```python
from build123d import *

# Parameters (mm, degrees)
SKETCH1_W           = 40
SKETCH1_H           = 40
BOSS_EXTRUDE1_DEPTH = 5
FILLET1_R           = 5
SKETCH2_R           = 15
BOSS_EXTRUDE2_DEPTH = 2.5
SKETCH3_R           = 3
BOSS_EXTRUDE3_DEPTH = 22.5
BOSS_EXTRUDE5_DEPTH = 82
CHAMFER1_SIZE       = 0.5
SKETCH5_R           = 2.15
CUT_EXTRUDE1_DEPTH  = 10
SKETCH6_W           = 8.611155486
SKETCH6_H           = 40
BOSS_EXTRUDE6_DEPTH = 12
CHAMFER2_SIZE       = 5


with BuildPart() as part:
    # Sketch1 → Boss-Extrude1 (new body)
    with BuildSketch(Plane.XY):
        Rectangle(SKETCH1_W, SKETCH1_H)
    extrude(amount=BOSS_EXTRUDE1_DEPTH)

    # Fillet1
    fillet1_edges = [part.edges().sort_by_distance(p)[0] for p in [
        (20, -20, 2.5),
        (-20, -20, 2.5),
        (-20, 20, 2.5),
        (20, 20, 2.5),
    ]]
    fillet(fillet1_edges, radius=FILLET1_R)

    # Sketch2 → Boss-Extrude2 (add)
    with BuildSketch(Plane.XY.offset(5)):
        Circle(SKETCH2_R)
    extrude(amount=BOSS_EXTRUDE2_DEPTH)

    # Sketch3 → Boss-Extrude3 (add)
    with BuildSketch(Plane.XY.offset(7.5)):
        with Locations(Location((0, 0, 0), (0, 0, 180))):
            Circle(SKETCH3_R)
    extrude(amount=BOSS_EXTRUDE3_DEPTH)

    # Sketch4 → Boss-Extrude5 (add)
    with BuildSketch(Plane(origin=(0, 0, 0), x_dir=(-1, 0, 0), z_dir=(0, 0, -1))):
        with BuildLine():
            Line((-20, -15), (-20, 15))
            ThreePointArc((-20, 15), (-18.535533906, 18.535533906), (-15, 20))
            Line((-15, 20), (15, 20))
            ThreePointArc((15, 20), (18.535533906, 18.535533906), (20, 15))
            Line((20, 15), (20, -15))
            ThreePointArc((20, -15), (18.535533906, -18.535533906), (15, -20))
            Line((15, -20), (-15, -20))
            ThreePointArc((-15, -20), (-18.535533906, -18.535533906), (-20, -15))
        make_face()
    extrude(amount=BOSS_EXTRUDE5_DEPTH)

    # Chamfer1
    chamfer1_edges = [part.edges().sort_by_distance(p)[0] for p in [
        (3, 0, 30),
    ]]
    chamfer(chamfer1_edges, length=CHAMFER1_SIZE)

    # Sketch5 → Cut-Extrude1 (cut)
    with BuildSketch(Plane.XY.offset(5)):
        with Locations((-16.263455967, 16.263455967)):
            Circle(SKETCH5_R)
        with Locations((16.263455967, 16.263455967)):
            Circle(SKETCH5_R)
        with Locations((16.263455967, -16.263455967)):
            Circle(SKETCH5_R)
        with Locations((-16.263455967, -16.263455967)):
            Circle(SKETCH5_R)
    extrude(amount=-CUT_EXTRUDE1_DEPTH, mode=Mode.SUBTRACT)

    # Sketch6 → Boss-Extrude6 (add)
    with BuildSketch(Plane(origin=(0, 20, 0), x_dir=(1, 0, 0), z_dir=(0, 1, 0))):
        with Locations((0, 60)):
            Rectangle(SKETCH6_W, SKETCH6_H)
    extrude(amount=BOSS_EXTRUDE6_DEPTH)

    # Chamfer2
    chamfer2_edges = [part.edges().sort_by_distance(p)[0] for p in [
        (0, 32, -40),
    ]]
    chamfer(chamfer2_edges, length=CHAMFER2_SIZE)


solid = part.part
```
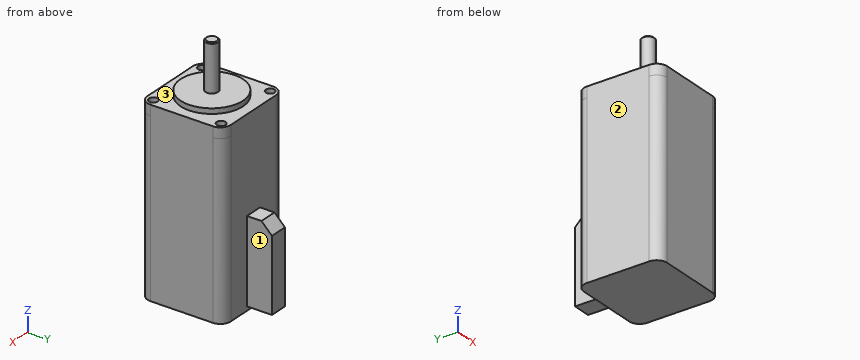
Here's how the part is built. I have some questions about the finished solid (model axes, mm). Face numbers are marked on the shaded views. A direction names the side the tool comes from. Give positions to 0.01 mm unless a question says otherwise; leave off trailing zeros. Order: outer loops, then holes, each group sorted by start corner. A loop starts at its lowest first (then second) coordinate and runs counter-clockwise, first axis right, second up. Notation, with made-up numbers: (-11, -34) - (40, -34) arc R17 ccw to (40, -11) - close; hole circle Ø11 at (13, 18.5). An arc over 180 degrees is marked (long way). Answer as a JSON object with one key per item and string values. Group by question number.
Item 1: For P1, Ø15, axis at x = -2.5, y = -5, coming from the +Z side; P2, Ø2, axis at x = 16.5, y = 17, coming from the +Z side; P3, Ø10, axis at x = 5, y = 7, coming from the +Z side; P4, Ø13, axis at y = 27, z = -63, coming from the +X side, each with a flat end and sliding along its axis, tell me the tip position at first contact or that it passes through.
Item 2: If we section it at A-A on z = -33: Please give me the cut outline in (x, y), and give its area (3 significant figures).
Item 3: Which directions (+Z, -Z, +X, -X, +Y, -Y) give clear straight access to the entire face, cutting with the end or side of a thin tool? Please do the marked faces 1, 2 and 3.
Item 4: If we section it at C-C on x = 0: Please give me the cut outline in (y, z).
Item 5: Please list where these lines run through material, in increasing order: probe 1 along Y at (x, z) = (14, -48.5); probe 2 along Z at (x, y) = (-1.5, 13); probe 3 along Y at (x, z) = (-3, -43).
Item 6: If we section it at D-D on z = -55: Please give me the cut outline in (x, y).
Item 7: If we section it at B-B on y = 0: Please give me the cut outline in (x, z).
Result set:
{
 "1": {"P1": "z = 30", "P2": "z = -5", "P3": "z = 7.5", "P4": "x = 4.31"},
 "2": {"outline": "(-20, -15) arc R5 ccw to (-15, -20) - (15, -20) arc R5 ccw to (20, -15) - (20, 15) arc R5 ccw to (15, 20) - (-15, 20) arc R5 ccw to (-20, 15) - close", "area": "1,580 mm²"},
 "3": {"face 1": "+Z, -Z, +X, +Y", "face 2": "+Z, -Z, -X, +Y, -Y", "face 3": "+Z"},
 "4": {"outline": "(-20, -82) - (20, -82) - (20, -80) - (32, -80) - (32, -45) - (27, -40) - (20, -40) - (20, 5) - (15, 5) - (15, 7.5) - (3, 7.5) - (3, 29.5) - (2.5, 30) - (-2.5, 30) - (-3, 29.5) - (-3, 7.5) - (-15, 7.5) - (-15, 5) - (-20, 5) - close"},
 "5": {"probe 1": "-20 to 20", "probe 2": "-82 to 7.5", "probe 3": "-20 to 30"},
 "6": {"outline": "(-20, -15) arc R5 ccw to (-15, -20) - (15, -20) arc R5 ccw to (20, -15) - (20, 15) arc R5 ccw to (15, 20) - (4.31, 20) - (4.31, 32) - (-4.31, 32) - (-4.31, 20) - (-15, 20) arc R5 ccw to (-20, 15) - close"},
 "7": {"outline": "(-20, -82) - (20, -82) - (20, 5) - (15, 5) - (15, 7.5) - (3, 7.5) - (3, 29.5) - (2.5, 30) - (-2.5, 30) - (-3, 29.5) - (-3, 7.5) - (-15, 7.5) - (-15, 5) - (-20, 5) - close"}
}
